The figure shows three views and two pictorial views of one solid part (mm, origin at its lowest corner). Answer the questions. A direction names the side the tool comes from. Give positions to 0.01 mm unless a question says otherwise; leave off trailing zeros. Write each loop counter-clockwise with the first axis right and the second up, starting at its lowest first coordinate (ties: lowest second). Pieces come first, ordered by that corner, then holes. Notation, with made-up numbers: (-39.75, 87.5) -> (-30.75, 87.5) arc R27 ccw to (-30.75, 105.5) -> close; hole circle Ø1 at (-16.75, 5.5). An arc over 180 degrees is marked (long way). Use a Markdown table: item, result.
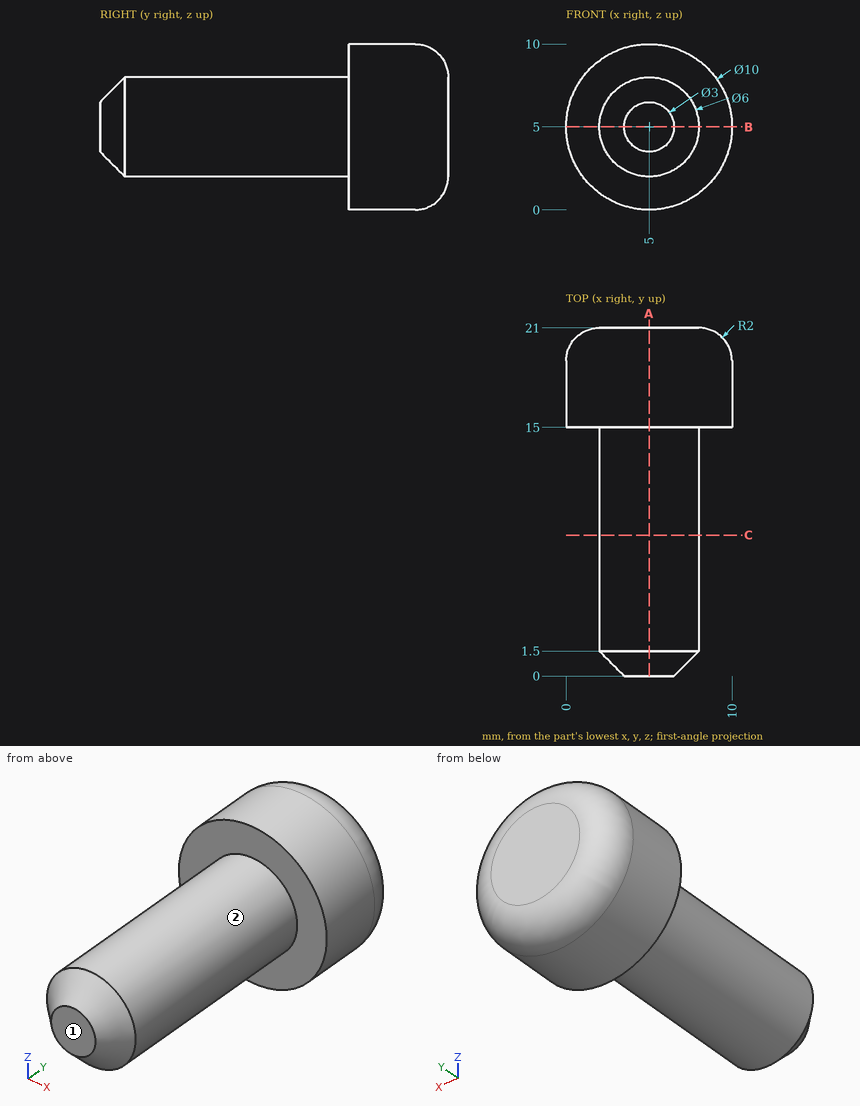
Item 1: A cutting plane is placed at B-B (z = 5). Give the vertices of the cut face in (x, y).
Return value:
| item | result |
|---|---|
| outline | (0, 15) -> (2, 15) -> (2, 1.5) -> (3.5, 0) -> (6.5, 0) -> (8, 1.5) -> (8, 15) -> (10, 15) -> (10, 19) arc R2 ccw to (8, 21) -> (2, 21) arc R2 ccw to (0, 19) -> close |
Item 2: Each of these flat-tipped pins is pushed along its axis until it touches: P1, Ø2, axis at x = 7, y = 11.5, coming from the -Z side; P2, Ø5, axis at y = 16, z = 4, coming from the -X side; P3, Ø6, axis at x = 1, z = 2.5, coming from the -Y side; P4, Ø5, axis at x = 7, z = 1.5, coming from the -Y side. Where does it stop, or does it pass through?
Return value:
| item | result |
|---|---|
| P1 | z = 2.17 |
| P2 | x = 0 |
| P3 | y = 0.22 |
| P4 | y = 0.03 |
Item 3: A cutting plane is placed at C-C (y = 8.5). Give the vertices of the cut face in (x, z).
Return value:
| item | result |
|---|---|
| outline | circle Ø6 at (5, 5) |
Item 4: A tool of negligible diameter and unlimited length cuts with its end or side. For the marked faces 1 and 2, from which of +Z, -Z, +X, -X, +Y, -Y can it reach the whole face along a straight path? Write none if from no direction.
Return value:
| item | result |
|---|---|
| face 1 | +Z, -Z, +X, -X, -Y |
| face 2 | -Y |
Item 5: A cutting plane is placed at A-A (x = 5). Give the vertices of the cut face in (y, z).
Return value:
| item | result |
|---|---|
| outline | (0, 3.5) -> (1.5, 2) -> (15, 2) -> (15, 0) -> (19, 0) arc R2 ccw to (21, 2) -> (21, 8) arc R2 ccw to (19, 10) -> (15, 10) -> (15, 8) -> (1.5, 8) -> (0, 6.5) -> close |
Item 6: Straight lines are drawn through the part: line 1 along Y through (x, z) = (7.5, 3.25); line 2 along Y through (x, z) = (1.5, 8); line 3 along X through (y, z) = (17, 8.75). For each, find the intervals that lie inside material, in ascending order. Write a range as [from, to].
Return value:
| item | result |
|---|---|
| line 1 | [15, 21] |
| line 2 | [15, 20.19] |
| line 3 | [1.69, 8.31] |
